from build123d import *

# Parameters (mm, degrees)
F0_W     = 450
F0_H     = 280
F1_DEPTH = 225
F2_T     = -12.7
F3_R     = 12.7
F4_DEPTH = 450.001
F5_W     = 450
F5_H     = 280
F6_DEPTH = 127
F7_W     = 424.6
F7_H     = 267.3
F8_DEPTH = 139.701


with BuildPart() as f1:
    # F0 (on Front) → F1 (new body, symmetric)
    with BuildSketch(Plane.XZ):
        with Locations((90.62104, -7.292895)):
            Rectangle(F0_W, F0_H)
    extrude(amount=F1_DEPTH, both=True)

    # F2
    f2_openings = [f1.faces().sort_by_distance(p)[0] for p in [
        (90.62104, 0, 132.707105),
    ]]
    offset(amount=F2_T, openings=f2_openings)

    # F3 (on face) → F4 (cut, through all)
    with BuildSketch(Plane.XZ.offset(225)):
        with Locations((100.62104, 40.667105)):
            Circle(F3_R)
    extrude(amount=-F4_DEPTH, mode=Mode.SUBTRACT)

    # F5 (on face) → F6 (join)
    with BuildSketch(Plane.YZ.offset(315.62104)):
        with Locations((0, -7.292895)):
            Rectangle(F5_W, F5_H)
    extrude(amount=F6_DEPTH)

    # F7 (on face) → F8 (cut, through all)
    with BuildSketch(Plane(origin=(302.92104, 0, 0), x_dir=(0, -1, 0), z_dir=(-1, 0, 0))):
        with Locations((0, -0.942895)):
            Rectangle(F7_W, F7_H)
    extrude(amount=-F8_DEPTH, mode=Mode.SUBTRACT)


solid = f1.part
Geometry check sheet. Reference: the model listing, model coordinates, mm. A direction names the side the tool comes from. Give positions to 0.01 mm unless a question says otherwise; leave off trailing zeros. Order: outer loops, then holes, each group sorted by start corner. A loop starts at its lowest first (then second) coordinate and runs counter-clockwise, first axis right, second up.
1) Cross-section at B-B (x = -44). Record the boundary of the cut face in (y, z), then the cut area to 3 significant figures.
Results are:
outline: (-225, -147.29) - (225, -147.29) - (225, 132.71) - (212.3, 132.71) - (212.3, -134.59) - (-212.3, -134.59) - (-212.3, 132.71) - (-225, 132.71) - close
area: 12,500 mm2
2) Cross-section at C-C (y = -119.5). Record the boundary of the cut face in (x, z), then the cut area to 3 significant figures.
Results are:
outline: (-134.38, -147.29) - (442.62, -147.29) - (442.62, -134.59) - (-121.68, -134.59) - (-121.68, 132.71) - (-134.38, 132.71) - close
area: 10,700 mm2
3) Gauge pin test, flat ends, axial feed: pin 1 (12 mm diameter, centred on y = -71, z = 100, fed in from +X); pin 2 (4 mm diameter, centred on x = 192.5, y = 100, fed in from +Z). Record the tip position at first contact, or that the pin passes through.
Results are:
pin 1: stops at x = -121.68
pin 2: stops at z = -134.59
4) Cross-section at A-A (z = -64.5). Record the boundary of the cut face in (x, y).
Results are:
outline: (-134.38, -225) - (442.62, -225) - (442.62, -212.3) - (-121.68, -212.3) - (-121.68, 212.3) - (442.62, 212.3) - (442.62, 225) - (-134.38, 225) - close
5) Draft check along Y on faces 3 (the cylindrical face through (91.26, -218.74, 49.25)), 4 (the flat face through (150, 225, -9)), 5 (the flat face through (157, 3, -134.593)). Enter one of: released by +Y, released by -Y, zero draft, split by the parting line, or undercut.
Results are:
face 3: zero draft
face 4: released by +Y
face 5: undercut
6) Material ranges on probe 1 along Y at (x, z) = (-49.5, 53); probe 2 along X at (y, z) = (39.5, 9.5); probe 3 along Z at (x, y) = (115, -86), recorded low to high.
Results are:
probe 1: y = -225 to -212.3, 212.3 to 225
probe 2: x = -134.38 to -121.68
probe 3: z = -147.29 to -134.59
7) Tool access check on faces 1 (the flat face through (-125, -1, 132.707)), 2 (the flat face through (157, 212.3, -3)). Record the directions out of +Z, -Z, +X, -X, +Y, -Y that give a thin tool (end or side, any length) a straight path to the whole face; none if there is none.
Results are:
face 1: +Z, +X, -X, +Y, -Y
face 2: +Z, +X
